from build123d import *

# Parameters (mm, degrees)
SKETCH1_R           = 27.5
SKETCH1_R_2         = 2.0193
BOSS_EXTRUDE1_DEPTH = 2.5
SKETCH2_R           = 17.46
BOSS_EXTRUDE2_DEPTH = 4
CHAMFER5_SIZE       = 1
SKETCH6_R           = 14
CUT_EXTRUDE1_DEPTH  = 10
SKETCH9_R           = 16
CUT_EXTRUDE2_DEPTH  = 2


with BuildPart() as part:
    # Sketch1 → Boss-Extrude1 (new body)
    with BuildSketch(Plane(origin=(0, 0, 0), x_dir=(0, 0, -1), z_dir=(1, 0, 0))):
        Circle(SKETCH1_R)
        with Locations((0, 20.64)):
            Circle(SKETCH1_R_2, mode=Mode.SUBTRACT)
        with Locations((17.874764334, 10.32)):
            Circle(SKETCH1_R_2, mode=Mode.SUBTRACT)
        with Locations((17.874764334, -10.32)):
            Circle(SKETCH1_R_2, mode=Mode.SUBTRACT)
        with Locations((0, -20.64)):
            Circle(SKETCH1_R_2, mode=Mode.SUBTRACT)
        with Locations((-17.874764334, -10.32)):
            Circle(SKETCH1_R_2, mode=Mode.SUBTRACT)
        with Locations((-17.874764334, 10.32)):
            Circle(SKETCH1_R_2, mode=Mode.SUBTRACT)
    extrude(amount=BOSS_EXTRUDE1_DEPTH)

    # Sketch2 → Boss-Extrude2 (add)
    with BuildSketch(Plane.ZY):
        with Locations(Location((0, 0, 0), (0, 0, 180))):
            Circle(SKETCH2_R)
    extrude(amount=BOSS_EXTRUDE2_DEPTH)

    # Chamfer5
    chamfer5_edges = [part.edges().sort_by_distance(p)[0] for p in [
        (-4, 0, 17.46),
    ]]
    chamfer(chamfer5_edges, length=CHAMFER5_SIZE)

    # Sketch6 → Cut-Extrude1 (cut)
    with BuildSketch(Plane(origin=(-4, 0, 0), x_dir=(0, 0, -1), z_dir=(1, 0, 0))):
        Circle(SKETCH6_R)
    extrude(amount=CUT_EXTRUDE1_DEPTH, mode=Mode.SUBTRACT)

    # Sketch9 → Cut-Extrude2 (cut)
    with BuildSketch(Plane(origin=(2.5, 0, 0), x_dir=(0, 0, -1), z_dir=(1, 0, 0))):
        Circle(SKETCH9_R)
    extrude(amount=-CUT_EXTRUDE2_DEPTH, mode=Mode.SUBTRACT)


solid = part.part
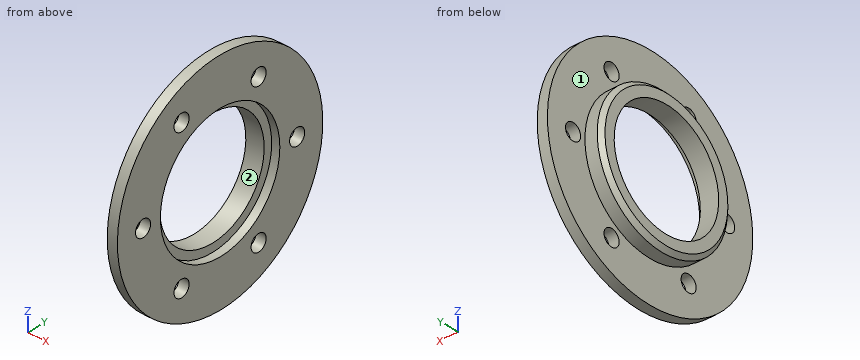
Could you check a few things on this model? Use its own coordinates, in mm. Face numbers are marked on the shaded views. A direction names the side the tool comes from. Give positions to 0.01 mm unless a question says otherwise; leave off trailing zeros. Write each loop counter-clockwise with the first axis right and the second up, starting at its lowest first coordinate (ties: lowest second). Pieces come first, ordered by that corner, then holes. Notation, with made-up numbers: (64.5, 50.25) -> (82.5, 50.25) arc R7 cw to (82.5, 61.25) -> close; hole circle Ø1 at (21, 81). An arc over 180 degrees is marked (long way). Answer as CSV lines item,"result". Start each with the question number.
(1) If we section it at C-C, the plane x = -1.75: Write out the boundary of the cut face in (y, z).
(2) Please list where these lines run through material, in increasing order: line 1 (Z direction, x = 0.75, y = -9.5); line 2 (Y direction, x = -3.5, z = 12.5); line 3 (Z direction, x = 0.5, y = 22).
(3) If we section it at B-B, the plane z = 18.5: Write out the boundary of the cut face in (x, y).
(4) If we section it at A-A, the plane y = 0: Write out the boundary of the cut face in (x, z), and give its area (3 significant figures).
(5) If we section it at D-D, the plane y = -19.5: Write out the boundary of the cut face in (x, z).
(6) I'm going to push flat-ended pins straight in: pin 1 Ø6.5 at (y, z) = (-20.64, 0) entering from +X; pin 2 Ø4.5 at (y, z) = (20.64, 0) entering from -X; pin 3 Ø3 at (x, z) = (1.5, 15.5) entering from +Y. Where does each tip first touch, or does it pass through?
(7) Which directions (+Z, -Z, +X, -X, +Y, -Y) give clear straight access to the entire face, cutting with the end or side of a thin tool? Please do the marked faces 1 and 2.
Answer list:
1,outline,"circle Ø34.92 at (0, 0); hole circle Ø28 at (0, 0)"
2,line 1,"-25.81 to -19.72, -16.03 to -12.87, 12.87 to 16.03, 19.72 to 25.81"
2,line 2,"-11.46 to -6.3, 6.3 to 11.46"
2,line 3,"-16.5 to -1.49, 1.49 to 16.5"
3,outline,"(0, -20.35) -> (2.5, -20.35) -> (2.5, -12.24) -> (0, -12.24) -> close; (0, -8.4) -> (2.5, -8.4) -> (2.5, 8.4) -> (0, 8.4) -> close; (0, 12.24) -> (2.5, 12.24) -> (2.5, 20.35) -> (0, 20.35) -> close"
4,outline,"(-4, -16.46) -> (-3, -17.46) -> (0, -17.46) -> (0, -27.5) -> (2.5, -27.5) -> (2.5, -16) -> (0.5, -16) -> (0.5, -14) -> (-4, -14) -> close; (-4, 14) -> (0.5, 14) -> (0.5, 16) -> (2.5, 16) -> (2.5, 27.5) -> (0, 27.5) -> (0, 17.46) -> (-3, 17.46) -> (-4, 16.46) -> close"
4,area,"86.2 mm^2"
5,outline,"(0, -19.39) -> (2.5, -19.39) -> (2.5, -1.67) -> (0, -1.67) -> close; (0, 1.67) -> (2.5, 1.67) -> (2.5, 19.39) -> (0, 19.39) -> close"
6,pin 1,"x = 2.5"
6,pin 2,"x = 0"
6,pin 3,"y = 23.67"
7,face 1,"-X"
7,face 2,"+X, -X"
